Geometry check sheet. Reference: the model listing, model coordinates, mm. A direction names the side the tool comes from. Give positions to 0.01 mm unless a question says otherwise; leave off trailing zeros. Loops run counter-clockwise (first coordinate to the right, second up) from the corner with the lowest first, then second, coordinate; pieces in that order, holes last.
1. Tool access check on faces 4 (the flat face through (-5, -6, 4.5)), 5 (the cylindrical face through (7.893, 9.233, 3.638)). Record the directions out of +Z, -Z, +X, -X, +Y, -Y that give a thin tool (end or side, any length) a straight path to the whole face; none if there is none.
2. Go/stop test with flat-tipped pins: pin 1 Ø8 at (x, y) = (-11.5, 7.5) entering from +Z; pin 2 Ø3 at (x, y) = (-19.5, 1) entering from +Z; pin 3 Ø1.5 at (y, z) = (3.5, 2.5) entering from -X; pin 4 Ø3.5 at (x, y) = (-19, 0) entering from -Z. Record where each tip stops, or that it passes through.
3. Cross-section at B-B, the plane x = 2. Record the cut outline in (y, z).
4. Material ranges on L1, parallel to Y at x = 2, z = 0.5; L2, parallel to Z at x = 2, y = -4.25; L3, parallel to X at y = -7, z = 4.15 (3 decimals), recorded low to high.
5. Cross-section at A-A, the plane y = 0. Record the cut outline in (x, z).
6. Cross-section at D-D, the plane x = -19. Record the cut outline in (y, z).
7. Release check for a two-part mould opening along Y. For faces 1 (the flat face through (8, -6, 4.5)), 2 (the conical face through (7.88, 9.31, 2.67)), 3 (the cylindrical face through (-9.05, -11.28, 0.41)) record: +Y half, -Y half, draft (parallel to the pull), parting line (faces both ways), or undercut.
Autodesk Inventor part; units mm, degrees
ref_plane "YZ Plane" through (0, 0, 0) normal (1, 0, 0) x (0, 1, 0)
ref_plane "XZ Plane" through (0, 0, 0) normal (0, 1, 0) x (-1, 0, 0)
ref_plane "XY Plane" through (0, 0, 0) normal (0, 0, 1) x (1, 0, 0)
sketch "Esquisse1" plane through (0, 0, 0) normal (0, 0, 1) x (1, 0, 0)
  line L0 (-9.1, 11.5) -> (13.9, 11.5)
  circle A0 centre (-19, 0) radius 3.1
  line L1 (-9.1, -11.5) -> (13.9, -11.5)
  line L2 (-9.1, -11.5) -> (-20.8866, -2.4598)
  arc A1 (13.9, -11.5) -> (13.9, 11.5) centre (1.4556, 0) ccw
  circle A2 centre (-19, 0) radius 2
  line L3 (-9.1, 11.5) -> (-20.8866, 2.4598)
  point P0 (0, 0)
  dimension "d0" = 6.2
  dimension "d1" = 23
  dimension "d2" = 23
  dimension "d3" = 23
  dimension "d4" = 11.5
  dimension "d5" = 11.5
  dimension "d6" = 9.9
  dimension "d7" = 9.9
  dimension "d8" = 19
  dimension "d9" = 40.5
  dimension "d10" = 4
extrude "Extrusion1" add sketch "Esquisse1" along normal blind 0.8
fillet "Congé1" radius 4 2 edges at (13.9, -11.5, 0.4) (13.9, 11.5, 0.4)
fillet "Congé2" radius 4 2 edges at (-9.1, 11.5, 0.4) (-9.1, -11.5, 0.4)
sketch "Esquisse3" plane through (0, 0, 0.8) normal (0, 0, 1) x (1, 0, 0)
  circle A0 centre (-19, 0) radius 2
  circle A1 centre (-19, 0) radius 3.1
  circle A2 centre (-19, 0) radius 2
  point P0 (0, 0)
  dimension "d16" = 4
  dimension "d17" = 6.2
extrude "Extrusion2" add sketch "Esquisse3" along normal blind 1
sketch "Esquisse4" plane through (0, 0, 0.8) normal (0, 0, 1) x (1, 0, 0)
  circle A0 centre (2, 0) radius 3
  line L0 (12.0058, 11.5) -> (-7.7427, 11.5)
  circle A1 centre (-19, 0) radius 2
  point P0 (0, 0)
  dimension "d20" = 6
  dimension "d21" = 11.5
  dimension "d22" = 21
extrude "Extrusion3" cut sketch "Esquisse4" against normal through all contours A0
sketch "Esquisse5" plane through (0, 0, 0.8) normal (0, 0, 1) x (1, 0, 0)
  circle A0 centre (-4.5, 6.5) radius 4
  circle A1 centre (8.5, 6.5) radius 4
  circle A2 centre (8.5, -6.5) radius 4
  circle A3 centre (-4.5, -6.5) radius 4
  circle A4 centre (2, 0) radius 3
  point P0 (0, 0)
  dimension "d25" = 8
  dimension "d26" = 8
  dimension "d27" = 8
  dimension "d28" = 8
  dimension "d29" = 13
  dimension "d30" = 13
  dimension "d31" = 6.5
  dimension "d32" = 6.5
  dimension "d34" = 6.5
  dimension "d35" = 6.5
  dimension "d36" = 13
  dimension "d37" = 6.5
extrude "Extrusion4" add sketch "Esquisse5" along normal blind 2 contours A0 | A1 | A2 | A3
sketch "Esquisse7" plane through (-4.5, 6.5, 2.8) normal (0, 0, 1) x (1, 0, 0)
  circle A0 centre (0, 0) radius 2.8
  circle A1 centre (13, 0) radius 2.8
  circle A2 centre (13, -13) radius 2.8
  circle A3 centre (0, -13) radius 2.8
  circle A4 centre (0, 0) radius 4
  circle A5 centre (13, 0) radius 4
  circle A6 centre (13, -13) radius 4
  circle A7 centre (0, -13) radius 4
  point P0 (4.5, -6.5)
  dimension "d49" = 5.6
  dimension "d50" = 5.6
  dimension "d51" = 5.6
  dimension "d52" = 5.6
extrude "Extrusion6" add sketch "Esquisse7" along normal blind 1.7 contours A0 | A1 | A2 | A3
chamfer "Chanfrein2" distance 1.2 distance2 2 1 edges at (-8.5, 6.5, 2.8) measured on face at (-0.9659, 5.9576, 2.8)
chamfer "Chanfrein3" distance 1.2 distance2 2 1 edges at (4.5, 6.5, 2.8) measured on face at (12.0613, 6.1809, 2.8)
chamfer "Chanfrein4" distance 1.2 distance2 2 1 edges at (-8.5, -6.5, 2.8) measured on face at (-0.9659, -7.0424, 2.8)
chamfer "Chanfrein5" distance 1.2 distance2 2 1 edges at (4.5, -6.5, 2.8) measured on face at (12.0341, -7.0424, 2.8)
equation "\"d3\" = d2"
equation "\"d5\" = d4"
equation "\"d26\" = d25"
equation "\"d27\" = d25"
equation "\"d28\" = d25"
equation "\"d30\" = d29"
equation "\"d31\" = 0.5 * d29"
equation "\"d32\" = d31"
equation "\"d34\" = d32"
equation "\"d35\" = d32"
equation "\"d36\" = d29"
equation "\"d37\" = d32"
equation "\"d50\" = d49"
equation "\"d51\" = d49"
equation "\"d52\" = d49"
properties part number "Membrane-DPAD" material "Caoutchouc"
Result:
1. face 4: +Z, +X, -X, +Y, -Y
1. face 5: +Z
2. pin 1: stops at z = 2.35
2. pin 2: stops at z = 1.8
2. pin 3: stops at x = -6.69
2. pin 4: passes through
3. outline: (-11.5, 0) - (-3, 0) - (-3, 0.8) - (-11.5, 0.8) - close; (3, 0) - (11.5, 0) - (11.5, 0.8) - (3, 0.8) - close
4. L1: y = -11.5 to -3, 3 to 11.5
4. L2: z = 0 to 0.8
4. L3: x = -7.255 to -1.745, 5.745 to 11.255
5. outline: (-22.1, 0) - (-21, 0) - (-21, 1.8) - (-22.1, 1.8) - close; (-17, 0) - (-1, 0) - (-1, 0.8) - (-15.9, 0.8) - (-15.9, 1.8) - (-17, 1.8) - close; (5, 0) - (18.4, 0) - (18.4, 0.8) - (5, 0.8) - close
6. outline: (-3.91, 0) - (-2, 0) - (-2, 1.8) - (-3.1, 1.8) - (-3.1, 0.8) - (-3.91, 0.8) - close; (2, 0) - (3.91, 0) - (3.91, 0.8) - (3.1, 0.8) - (3.1, 1.8) - (2, 1.8) - close
7. face 1: draft
7. face 2: undercut
7. face 3: -Y half
